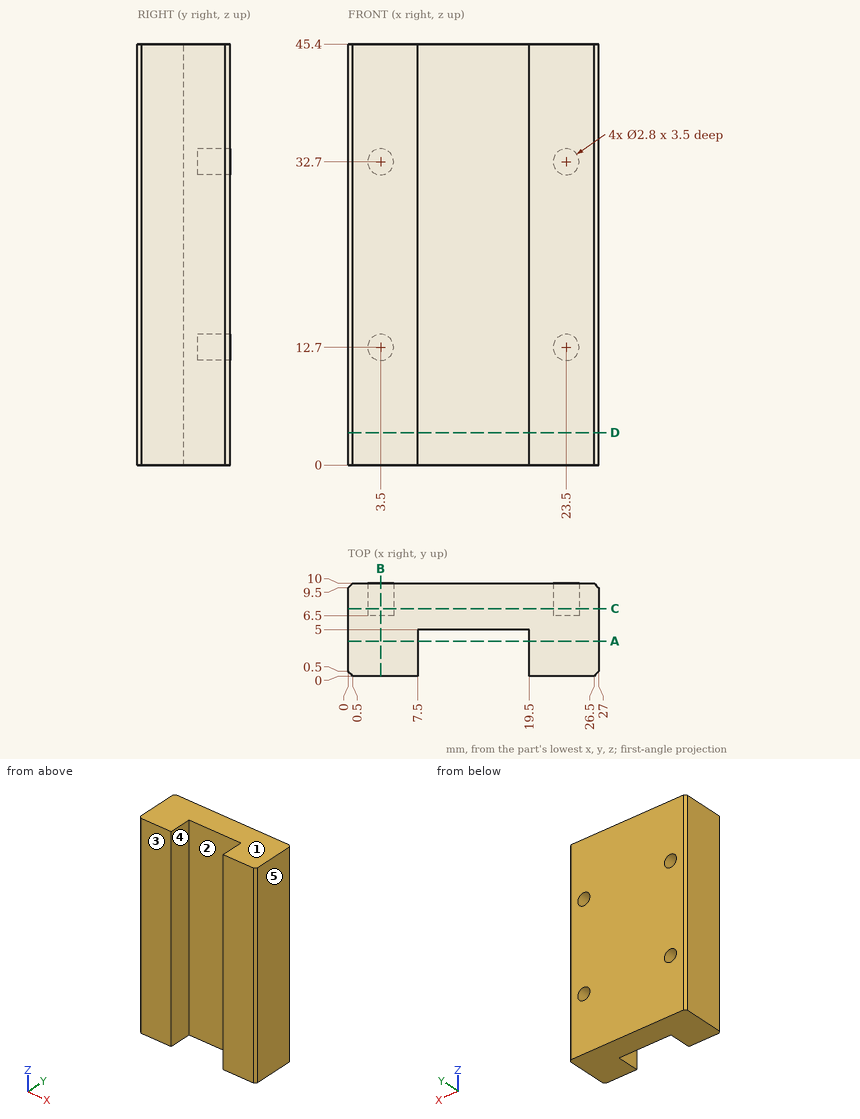
Verification items for this drawing (mm, ordinates from the low corner). A direction names the side the tool comes from. Coordinates: 2 decimals unless noted, no trailing zeros. Loops run counter-clockwise (first coordinate to the right, second up) from the corner with the lowest first, then second, coordinate; pieces in that order, holes last. Notation, with made-up numbers: (4.25, -34) -> (11.25, -34) arc R30 cw to (11.25, 1) -> close; hole circle Ø5 at (-34, 17). An arc over 180 degrees is marked (long way). Answer in a Markdown table with one row per item. Add a question column.
1. Depth check by flat-ended pin: P1, Ø1.7, axis at x = 23.5, z = 32.7, coming from the -Y side; P2, Ø1.5, axis at x = 10.5, z = 25.5, coming from the -Y side; P3, Ø0.8, axis at x = 3.5, z = 33, coming from the +Y side. Enter the tip coordinate at first touch or a pass-through.
2. Section check D-D, the plane z = 3.5. Enter the section's corners in (x, y).
3. Section check C-C, the plane y = 7.25. Enter the section's corners in (x, z).
4. Draft check along X on the marked faces 3, 4 and 5. Enter one of: +X half, -X half, draft (parallel to the pull), parting line (faces both ways), or undercut.
5. Section check A-A, the plane y = 3.75. Enter the section's corners in (x, z), then the cut area to 3 significant figures.
6. Access from +Z, -Z, +X, -X, +Y, -Y to the whole of each face (thin tool, end or side, straight path). Record for the marked faces 1 and 2.
7. Material ranges on probe 1 along X at (y, z) = (9.1, 12.7); probe 2 along X at (y, z) = (1, 22.5); probe 3 along Y at (x, z) = (11.5, 35.5), recorded low to high. Write a range as [from, to].
8. Section check B-B, the plane x = 3.5. Enter the section's corners in (y, z).
Derived:
| question | item | result |
|---|---|---|
| 1 | P1 | stops at y = 0 |
| 1 | P2 | stops at y = 5 |
| 1 | P3 | stops at y = 6.5 |
| 2 | outline | (0, 0.5) -> (0.5, 0) -> (7.5, 0) -> (7.5, 5) -> (19.5, 5) -> (19.5, 0) -> (26.5, 0) -> (27, 0.5) -> (27, 9.5) -> (26.5, 10) -> (0.5, 10) -> (0, 9.5) -> close |
| 3 | outline | (0, 0) -> (27, 0) -> (27, 45.4) -> (0, 45.4) -> close; hole circle Ø2.8 at (3.5, 12.7); hole circle Ø2.8 at (3.5, 32.7); hole circle Ø2.8 at (23.5, 12.7); hole circle Ø2.8 at (23.5, 32.7) |
| 4 | face 3 | draft |
| 4 | face 4 | undercut |
| 4 | face 5 | +X half |
| 5 | outline | (0, 0) -> (7.5, 0) -> (7.5, 45.4) -> (0, 45.4) -> close; (19.5, 0) -> (27, 0) -> (27, 45.4) -> (19.5, 45.4) -> close |
| 5 | area | 681 mm² |
| 6 | face 1 | +Z, +X, -X, +Y, -Y |
| 6 | face 2 | +Z, -Z, -Y |
| 7 | probe 1 | x = [0, 2.1], [4.9, 22.1], [24.9, 27] |
| 7 | probe 2 | x = [0, 7.5], [19.5, 27] |
| 7 | probe 3 | y = [5, 10] |
| 8 | outline | (0, 0) -> (10, 0) -> (10, 11.3) -> (6.5, 11.3) -> (6.5, 14.1) -> (10, 14.1) -> (10, 31.3) -> (6.5, 31.3) -> (6.5, 34.1) -> (10, 34.1) -> (10, 45.4) -> (0, 45.4) -> close |
